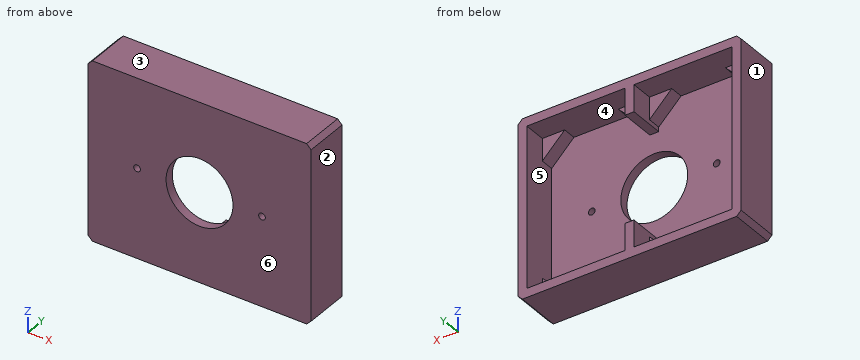
```python
from build123d import *

# Parameters (mm, degrees)
SKETCH1_W           = 100
SKETCH1_H           = 80
BOSS_EXTRUDE1_DEPTH = 20
SHELL2_T            = -4
SKETCH14_W          = 4
SKETCH14_H          = 12
BOSS_EXTRUDE5_DEPTH = 16
SKETCH5_R           = 15
CUT_EXTRUDE1_DEPTH  = 5
BOSS_EXTRUDE6_DEPTH = 6
CHAMFER1_SIZE       = 2
SKETCH16_R          = 1.5
CUT_EXTRUDE2_DEPTH  = 4


with BuildPart() as part:
    # Sketch1 → Boss-Extrude1 (new body)
    with BuildSketch(Plane(origin=(0, 0, 0), x_dir=(1, 0, 0), z_dir=(0, 1, 0))):
        Rectangle(SKETCH1_W, SKETCH1_H)
    extrude(amount=-BOSS_EXTRUDE1_DEPTH)

    # Shell2
    shell2_openings = [part.faces().sort_by_distance(p)[0] for p in [
        (0, 0, 0),
    ]]
    offset(amount=SHELL2_T, openings=shell2_openings, kind=Kind.INTERSECTION)

    # Sketch14 → Boss-Extrude5 (add)
    with BuildSketch(Plane(origin=(0, 0, 0), x_dir=(1, 0, 0), z_dir=(0, 1, 0))):
        with Locations((0, -30)):
            Rectangle(SKETCH14_W, SKETCH14_H)
        with Locations((0, 30)):
            Rectangle(SKETCH14_W, SKETCH14_H)
    extrude(amount=-BOSS_EXTRUDE5_DEPTH)

    # Sketch5 → Cut-Extrude1 (cut, through all)
    with BuildSketch(Plane(origin=(0, -16, 0), x_dir=(1, 0, 0), z_dir=(0, 1, 0))):
        Circle(SKETCH5_R)
    extrude(amount=-CUT_EXTRUDE1_DEPTH, mode=Mode.SUBTRACT)

    # Sketch15 → Boss-Extrude6 (add)
    with BuildSketch(Plane(origin=(0, -16, 0), x_dir=(1, 0, 0), z_dir=(0, 1, 0))):
        Polygon((-46, 36), (-46, 26), (-36, 36), align=None)
        Polygon((-2, 36), (-2, 26), (-12, 36), align=None)
        Polygon((-2, -26), (-12, -36), (-2, -36), align=None)
        Polygon((-46, -26), (-36, -36), (-46, -36), align=None)
        Polygon((2, -36), (2, -26), (12, -36), align=None)
        Polygon((46, -36), (46, -26), (36, -36), align=None)
        Polygon((2, 26), (12, 36), (2, 36), align=None)
        Polygon((46, 26), (36, 36), (46, 36), align=None)
    extrude(amount=BOSS_EXTRUDE6_DEPTH)

    # Chamfer1
    chamfer1_edges = [part.edges().sort_by_distance(p)[0] for p in [
        (-50, -10, -40),
        (50, -10, -40),
        (50, -10, 40),
        (-50, -10, 40),
    ]]
    chamfer(chamfer1_edges, length=CHAMFER1_SIZE)

    # Sketch16 → Cut-Extrude2 (cut)
    with BuildSketch(Plane(origin=(0, -16, 0), x_dir=(1, 0, 0), z_dir=(0, 1, 0))):
        with Locations((-28, 0)):
            Circle(SKETCH16_R)
        with Locations((28, 0)):
            Circle(SKETCH16_R)
    extrude(amount=-CUT_EXTRUDE2_DEPTH, mode=Mode.SUBTRACT)


solid = part.part
```
The model under review builds one solid part; all positions refer to its coordinate system, in mm. Face numbers are marked on the shaded views. A direction names the side the tool comes from. Round coordinates to 2 decimals unless told otherwise and drop trailing zeros. Loops run counter-clockwise (first coordinate to the right, second up) from the corner with the lowest first, then second, coordinate; pieces in that order, holes last.
Item 1: Mouldability with a two-part tool opening along X and no side actions: class the marked faces 1, 2, 3 and 4 as released by +X, released by -X, zero draft, split by the parting line, or undercut.
Determined:
face 1: released by -X
face 2: released by +X
face 3: zero draft
face 4: undercut
Item 2: Take a section at A-A (x = 28). Write out the cut boundary in (y, z), then the cut area to 3 significant figures.
Determined:
outline: (-20, -40) - (0, -40) - (0, -36) - (-16, -36) - (-16, -1.5) - (-20, -1.5) - close; (-20, 1.5) - (-16, 1.5) - (-16, 36) - (0, 36) - (0, 40) - (-20, 40) - close
area: 436 mm2
Item 3: Take a section at C-C (y = -8.75). Write out the cut boundary in (x, z), then the cut area to 3 significant figures.
Determined:
outline: (-50, -38) - (-48, -40) - (48, -40) - (50, -38) - (50, 38) - (48, 40) - (-48, 40) - (-50, 38) - close; hole (-46, -36) - (-2, -36) - (-2, -24) - (2, -24) - (2, -36) - (46, -36) - (46, 36) - (2, 36) - (2, 24) - (-2, 24) - (-2, 36) - (-46, 36) - close
area: 1,460 mm2
Item 4: For line 1 (X direction, y = -7.75, z = -29.5); line 2 (X direction, y = -17.55, z = 0); line 3 (X direction, y = -0.75, z = -13.5), list the stretches that pass through material, from the lowest coordinate up.
Determined:
line 1: x = -50 to -46, -2 to 2, 46 to 50
line 2: x = -50 to -29.5, -26.5 to -15, 15 to 26.5, 29.5 to 50
line 3: x = -50 to -46, 46 to 50
Item 5: Clearance check with flat-ended pins moving along their axes: pin 1 Ø5 at (x, z) = (43, -29) entering from +Y; pin 2 Ø12 at (x, z) = (18, -21) entering from +Y. State where each tip first meets the part, or that it passes through.
Determined:
pin 1: stops at y = -10
pin 2: stops at y = -16
Item 6: For the marked faces 5 and 6, list the 3-axis set-ups (+Z, -Z, +X, -X, +Y, -Y) from which the entire face can be reached by the end or side of a thin tool; tool diameter is ignored.
Determined:
face 5: +Y
face 6: +Z, -Z, +X, -X, -Y
Item 7: Take a section at B-B (z = 0). Write out the cut boundary in (x, y), then the cut area to 3 significant figures.
Determined:
outline: (-50, -20) - (-29.5, -20) - (-29.5, -16) - (-46, -16) - (-46, 0) - (-50, 0) - close; (-26.5, -20) - (-15, -20) - (-15, -16) - (-26.5, -16) - close; (15, -20) - (26.5, -20) - (26.5, -16) - (15, -16) - close; (29.5, -20) - (50, -20) - (50, 0) - (46, 0) - (46, -16) - (29.5, -16) - close
area: 384 mm2
Item 8: Take a section at D-D (z = 12.5). Write out the cut boundary in (x, y), then the cut area to 3 significant figures.
Determined:
outline: (-50, -20) - (-8.29, -20) - (-8.29, -16) - (-46, -16) - (-46, 0) - (-50, 0) - close; (8.29, -20) - (50, -20) - (50, 0) - (46, 0) - (46, -16) - (8.29, -16) - close
area: 462 mm2
